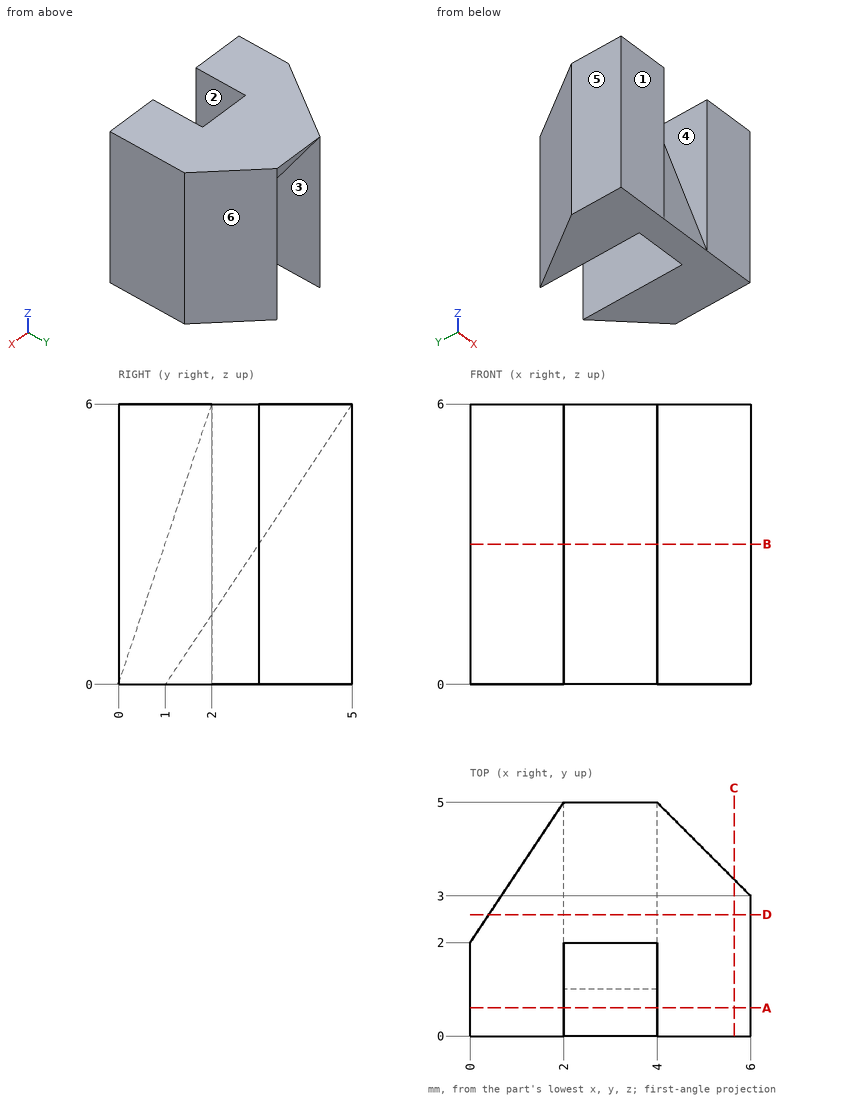
The figure shows three views and two pictorial views of one solid part (mm, origin at its lowest corner). Answer the questions. A direction names the side the tool comes from. Coordinates: 2 decimals unless noted, no trailing zeros. Order: outer loops, then holes, each group sorted by start corner. A loop starts at its lowest first (then second) coordinate and runs counter-clockwise, first axis right, second up.
Q1. Given P1, Ø2, axis at y = 1, z = 4, coming from the -X side; P2, Ø1.2, axis at y = 3.5, z = 4, coming from the -X side, each flat-ended and moving along its own axis, determine where each tip first touches the part or whether it passes through.
Q2. A cutting plane is placed at B-B, the plane z = 3. Write down the section's boundary in (x, y).
Q3. For a pull along X with two mould halves and no side action, classify the marked faces 4, 5 and 6 as pulls with the +X half, pulls with the -X half, needs draft (parallel to the pull), parting line crosses it, or undercut.
Q4. Which of the six approach directions +Z, -Z, +X, -X, +Y, -Y give full straight-line access (tool end or side, diameter ignored) to the marked faces 1, 2 and 3?
Q5. A cutting plane is placed at D-D, the plane y = 2.6. Write down the section's boundary in (x, z), and give its area (3 significant figures).
Q6. Consider line 1 (X direction, y = 0.75, z = 3.5); line 2 (X direction, y = 3.1, z = 2.25); line 3 (Y direction, x = 3.7, z = 3). Determine where each line is inside the solid, lowest interval first.
Q7. A cutting plane is placed at A-A, the plane y = 0.6. Write down the section's boundary in (x, z), and give its area (3 significant figures).
Q8. A cutting plane is placed at C-C, the plane x = 5.65. Write down the section's boundary in (y, z).
Answers follow:
1. P1: stops at x = 0
1. P2: stops at x = 0.6
2. outline: (0, 0) - (2, 0) - (2, 1) - (4, 1) - (4, 0) - (6, 0) - (6, 3) - (4, 5) - (4, 3) - (2, 3) - (2, 5) - (0, 2) - close
3. face 4: undercut
3. face 5: pulls with the -X half
3. face 6: pulls with the +X half
4. face 1: +Z, -Z, +X, -X, -Y
4. face 2: +Z, -Y
4. face 3: -Z, +Y
5. outline: (0.4, 0) - (2, 0) - (2, 2.4) - (4, 2.4) - (4, 0) - (6, 0) - (6, 6) - (0.4, 6) - close
5. area: 28.8 mm2
6. line 1: x = 0 to 2, 4 to 6
6. line 2: x = 0.73 to 2, 4 to 5.9
6. line 3: y = 1 to 3
7. outline: (0, 0) - (6, 0) - (6, 6) - (4, 6) - (4, 1.8) - (2, 1.8) - (2, 6) - (0, 6) - close
7. area: 27.6 mm2
8. outline: (0, 0) - (3.35, 0) - (3.35, 6) - (0, 6) - close
